Check sheet for the drawn part. Datum: minimum x, y, z corner. Units: mm. Coordinates: 2 decimals unless noted, no trailing zeros. Loops run counter-clockwise (first coordinate to the right, second up) from the corner with the lowest first, then second, coordinate; pieces in that order, holes last.
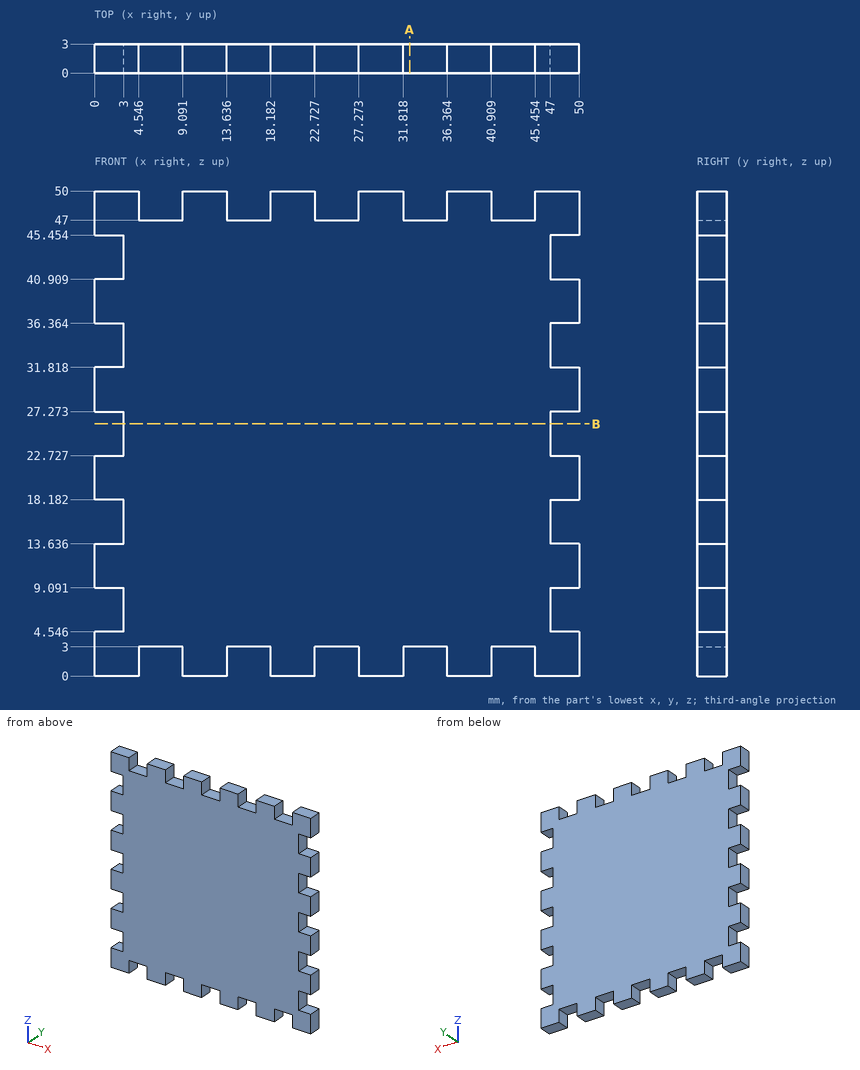
1) Scan lines: line 1 (Z direction, x = 47.5, y = 1.75) (1 decimal); line 2 (Z direction, x = 44, y = 0.4). Record each from-to range of solid material in increasing order.
Answer sheet:
line 1: z = 0 to 4.5, 9.1 to 13.6, 18.2 to 22.7, 27.3 to 31.8, 36.4 to 40.9, 45.5 to 50
line 2: z = 3 to 47
2) Section check A-A on x = 32.5. Enter the section's corners in (y, z).
Answer sheet:
outline: (0, 3) - (3, 3) - (3, 47) - (0, 47) - close
3) Depth check by flat-ended pin: pin 1 (1.5 mm diameter, centred on x = 33.5, y = 2, fed in from -Z). Enter the tip coordinate at first touch or a pass-through.
Answer sheet:
pin 1: stops at z = 3
4) Section check B-B on z = 26. Enter the section's corners in (x, y).
Answer sheet:
outline: (3, 0) - (47, 0) - (47, 3) - (3, 3) - close
